Autodesk Inventor part; units mm, degrees
ref_plane "YZ Plane" through (0, 0, 0) normal (1, 0, 0) x (0, 1, 0)
ref_plane "XZ Plane" through (0, 0, 0) normal (0, 1, 0) x (-1, 0, 0)
ref_plane "XY Plane" through (0, 0, 0) normal (0, 0, 1) x (1, 0, 0)
sketch "Skizze1" plane through (0, 0, 0) normal (0, 0, 1) x (1, 0, 0)
  circle A0 centre (0, 0) radius 20
  dimension "d0" = 40
extrude "Extrusion1" add sketch "Skizze1" along normal blind 20
fillet "Rundung1" radius 2 1 edges at (-20, 0, 20)
sketch "Skizze2" plane through (0, 0, 20) normal (0, 0, 1) x (1, 0, 0)
  circle A0 centre (10, 8) radius 3.75
  point P0 (0, 0)
  dimension "d4" = 7.5
hole "Bohrung1" at (10, 8, 20) direction (0, 0, -1) diameter 5 end through all
sketch "Skizze3" plane through (0, 0, 0) normal (0, 0, -1) x (-1, 0, 0)
  circle A0 centre (0, 0) radius 2.5
  circle A1 centre (0, 0) radius 2
  dimension "d12" = 5
  dimension "d13" = 4
extrude "Extrusion2" cut sketch "Skizze3" against normal blind 0.5
properties part number "Hub" material "ABS-Kunststoff"
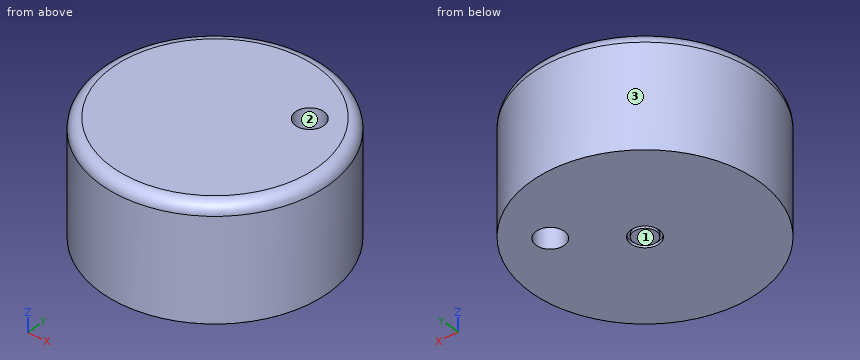
Could you check a few things on this model? Use its own coordinates, in mm. Face numbers are marked on the shaded views. Give positions to 0.01 mm unless a question says otherwise; leave off trailing zeros. Loops run counter-clockwise (first coordinate to the right, second up) from the corner with the lowest first, then second, coordinate; pieces in that order, holes last. Notation, with made-up numbers: (-23, 37.5) - (29, 37.5) arc R13 ccw to (29, 55.5) - close; hole circle Ø9 at (34, 62). An arc over 180 degrees is marked (long way). Use one line per item in the form item = value.
1. I'm going to push flat-ended pins straight in: pin 1 Ø5 at (x, z) = (0, 11) entering from -Y; pin 2 Ø4 at (y, z) = (-9.5, 11) entering from -X; pin 3 Ø1.5 at (x, y) = (0, -1) entering from -Z; pin 4 Ø1 at (x, z) = (-6.5, 9) entering from +Y. Where does each tip first touch, or does it pass through?
Response values:
pin_1 = -20
pin_2 = -18.54
pin_3 = 0
pin_4 = 19.08
2. Thinking about a two-plate mould opening in Y: for the marked faces 1, 2 and 3, which applies, released by +Y, released by -Y, zero draft, split by the parting line, or undercut?
Response values:
face_1 = zero draft
face_2 = undercut
face_3 = split by the parting line
3. I need wall thicknesses on probe 1 along Y at (x, z) = (0, 0.2); probe 2 along X at (y, z) = (9.5, 11.5); probe 3 along X at (y, z) = (8, 6.25). Which ranges of each line are inside material? Lowest first, please.
Response values:
probe_1 = -20 to -2.5, -2 to 2, 2.5 to 20
probe_2 = -17.6 to 8, 12 to 17.6
probe_3 = -18.33 to 7.5, 12.5 to 18.33
4. I want a section at A-A (z = 7.5). Please give me the cut outline in (x, y), and give its area (3 significant figures).
Response values:
outline = circle Ø40 at (0, 0); hole circle Ø5 at (10, 8)
area = 1,240 mm²
